Part model, mm, in its own coordinate system. A direction names the side the tool comes from. Round coordinates to 2 decimals unless told otherwise and drop trailing zeros. Write each loop counter-clockwise with the first axis right and the second up, starting at its lowest first coordinate (ties: lowest second). Pieces come first, ordered by that corner, then holes. Notation, with made-up numbers: (49, 77.25) -> (80, 77.25) arc R14 cw to (80, 97.25) -> close; hole circle Ø2 at (32, 48.5). An arc over 180 degrees is marked (long way). Return JSON: item names as keys, results as strings. Group by question number.
(1) Mould opens along Z. For faces 5 (the flat face through (-1, 1, 7)), 6 (the flat face through (-1, -1, -7)), 7 (the flat face through (51.5, -1, 0)) say: +Z half, -Z half, draft (parallel to the pull), parting line (faces both ways), or undercut.
(2) Saw through at A-A (x = 12.5). List the corners of the cut face in (y, z), plus the area to 3 significant figures.
(3) Saw through at B-B (y = 36). List the corners of the cut face in (x, z).
(4) Tool access for faces 1 (the cylindrical face through (-50.07, -45, 0.08)), 2 (the cylindrical face through (50, -45.07, 0.08)), 3 (the flat face through (-51.5, 1, 0)), 4 (the flat face through (0, 47, 6)): list every direction of +Z, -Z, +X, -X, +Y, -Y with a clear straight run to the whole face (end or side of a thin tool).
(5) Saw through at C-C (z = -1.5). List the corners of the cut face in (x, y).
(6) Drop flat-ended pins along their axis: pin 1 Ø3.5 at (y, z) = (-17.5, 2) entering from -X; pin 2 Ø3.5 at (y, z) = (-9, -2) entering from +X. Give the stop position or say it passes through.
(7) Drill centre lines: L1, parallel to Z at x = 52, y = -43; L2, parallel to X at y = 37.5, z = 2.25; L3, parallel to Y at x = 29.5, z = -4. Where is each one in solid material? Low to high. Write a range as from..to.
from build123d import *

# Parameters (mm, degrees)
PAD_DEPTH    = 6
PAD001_DEPTH = 1
PAD002_DEPTH = 1
FILLET_R     = 0.9


with BuildPart() as part:
    # Sketch → Pad (new body, symmetric)
    with BuildSketch(Plane.XY):
        with BuildLine():
            Line((-46.5, -46.5), (46.5, -46.5))
            ThreePointArc((46.5, -46.5), (50.035534, -45.035534), (51.5, -41.5))
            Line((51.5, -41.5), (51.5, 41.5))
            ThreePointArc((51.5, 41.5), (50.035534, 45.035534), (46.5, 46.5))
            Line((46.5, 46.5), (-46.5, 46.5))
            ThreePointArc((-46.5, 46.5), (-50.035534, 45.035534), (-51.5, 41.5))
            Line((-51.5, 41.5), (-51.5, -41.5))
            ThreePointArc((-51.5, -41.5), (-50.035534, -45.035534), (-46.5, -46.5))
        make_face()
    extrude(amount=PAD_DEPTH, both=True)

    # Sketch001 (on Face10 of Pad) → Pad001 (join)
    with BuildSketch(Plane.XY.offset(6)):
        with BuildLine():
            Line((-47.5, -52.5), (47.5, -52.5))
            ThreePointArc((47.5, -52.5), (54.571068, -49.571068), (57.5, -42.5))
            Line((57.5, -42.5), (57.5, 42.5))
            ThreePointArc((57.5, 42.5), (54.571068, 49.571068), (47.5, 52.5))
            Line((47.5, 52.5), (-47.5, 52.5))
            ThreePointArc((-47.5, 52.5), (-54.571068, 49.571068), (-57.5, 42.5))
            Line((-57.5, 42.5), (-57.5, -42.5))
            ThreePointArc((-57.5, -42.5), (-54.571068, -49.571068), (-47.5, -52.5))
        make_face()
    extrude(amount=PAD001_DEPTH)

    # Sketch002 (on Face4 of Pad001) → Pad002 (join)
    with BuildSketch(Plane(origin=(0, 0, -6), x_dir=(1, 0, 0), z_dir=(0, 0, -1))):
        with BuildLine():
            Line((-47.5, -52.5), (47.5, -52.5))
            ThreePointArc((47.5, -52.5), (54.571068, -49.571068), (57.5, -42.5))
            Line((57.5, -42.5), (57.5, 42.5))
            ThreePointArc((57.5, 42.5), (54.571068, 49.571068), (47.5, 52.5))
            Line((47.5, 52.5), (-47.5, 52.5))
            ThreePointArc((-47.5, 52.5), (-54.571068, 49.571068), (-57.5, 42.5))
            Line((-57.5, 42.5), (-57.5, -42.5))
            ThreePointArc((-57.5, -42.5), (-54.571068, -49.571068), (-47.5, -52.5))
        make_face()
    extrude(amount=PAD002_DEPTH)

    # Fillet
    fillet_edges = [part.edges().sort_by_distance(p)[0] for p in [
        (57.5, 0, -7),
        (57.5, 0, 7),
    ]]
    fillet(fillet_edges, radius=FILLET_R)


solid = part.part
Computed values:
{
 "1": {"face 5": "+Z half", "face 6": "-Z half", "face 7": "undercut"},
 "2": {"outline": "(-52.5, -6.1) arc R0.9 ccw to (-51.6, -7) -> (51.6, -7) arc R0.9 ccw to (52.5, -6.1) -> (52.5, -6) -> (46.5, -6) -> (46.5, 6) -> (52.5, 6) -> (52.5, 6.1) arc R0.9 ccw to (51.6, 7) -> (-51.6, 7) arc R0.9 ccw to (-52.5, 6.1) -> (-52.5, 6) -> (-46.5, 6) -> (-46.5, -6) -> (-52.5, -6) -> close", "area": "1,330 mm2"},
 "3": {"outline": "(-57.5, -6.1) arc R0.9 ccw to (-56.6, -7) -> (56.6, -7) arc R0.9 ccw to (57.5, -6.1) -> (57.5, -6) -> (51.5, -6) -> (51.5, 6) -> (57.5, 6) -> (57.5, 6.1) arc R0.9 ccw to (56.6, 7) -> (-56.6, 7) arc R0.9 ccw to (-57.5, 6.1) -> (-57.5, 6) -> (-51.5, 6) -> (-51.5, -6) -> (-57.5, -6) -> close"},
 "4": {"face 1": "-X, -Y", "face 2": "+X, -Y", "face 3": "-X, +Y, -Y", "face 4": "none"},
 "5": {"outline": "(-51.5, -41.5) arc R5 ccw to (-46.5, -46.5) -> (46.5, -46.5) arc R5 ccw to (51.5, -41.5) -> (51.5, 41.5) arc R5 ccw to (46.5, 46.5) -> (-46.5, 46.5) arc R5 ccw to (-51.5, 41.5) -> close"},
 "6": {"pin 1": "x = -51.5", "pin 2": "x = 51.5"},
 "7": {"L1": "-7..-6, 6..7", "L2": "-51.5..51.5", "L3": "-46.5..46.5"}
}
